Answer from the drawing. Dimensions are ordinates in mm from the lowest x, y and z of the part. A direction names the side the tool comes from. Coordinates: 2 decimals unless noted, no trailing zeros. Order: outer loops, then holes, each group sorted by start corner. A loop starts at its lowest first (then second) coordinate and runs counter-clockwise, first axis right, second up. Notation, with made-up numbers: (15.25, 30) - (66.25, 30) arc R14 cw to (66.25, 46) - close; hole circle Ø5 at (-22.5, 71.5). An arc over 180 degrees is marked (long way). Use a Markdown table: item, result. Add a question column.
Item 1: The part is cut by section A-A, the plane x = 60. Give the vertices of the cut face in (y, z) (1 decimal), then the cut area to 3 significant figures.
Item 2: The part is cut by section C-C, the plane z = 29.5. Give the vertices of the cut face in (x, y) (1 decimal).
Item 3: For the marked faces 1 and 2, determine the directions among +Z, -Z, +X, -X, +Y, -Y from which every point of the face is accessible in a straight line to the end or side of a thin tool.
Item 4: Find the intervals of material crossed by line 1 along Z through (x, y) = (42, 24); line 2 along Y through (x, z) = (83, 39.5) (1 decimal); line 3 along Y through (x, z) = (68.5, 32) (1 decimal), in increasing order.
Item 5: The part is cut by section D-D, the plane y = 98. Give the vertices of the cut face in (x, z), then the cut area to 3 significant figures.
Item 6: The part is cut by section B-B, the plane y = 57.5. Give the vertices of the cut face in (x, z).
Item 7: Flat-ended cylindrical pins translate along their axes: P1, Ø1, axis at x = 36, y = 64, coming from the -Z side; P2, Ø8, axis at x = 20, y = 32.5, coming from the +Z side. Find the tip coordinate at first contact, or state that the pin passes through.
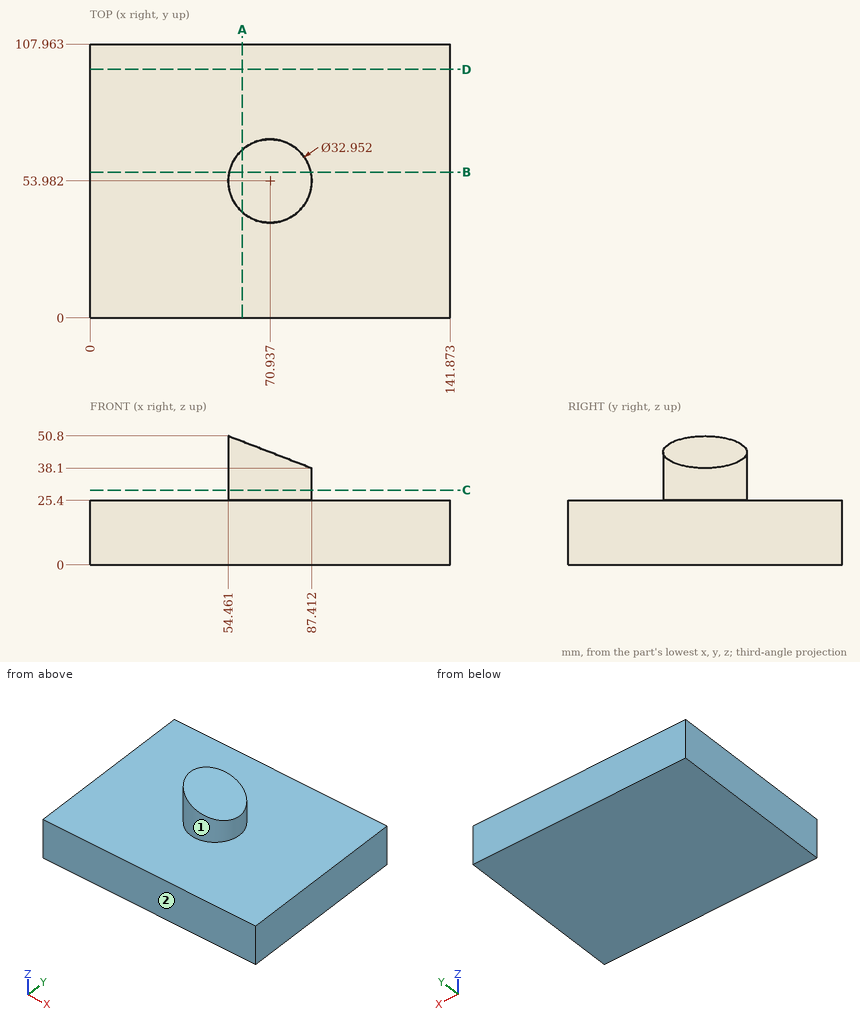
Solution:
| question | item | result |
|---|---|---|
| 1 | outline | (0, 0) - (108, 0) - (108, 25.4) - (66.3, 25.4) - (66.3, 48.7) - (41.7, 48.7) - (41.7, 25.4) - (0, 25.4) - close |
| 1 | area | 3,320 mm2 |
| 2 | outline | circle Ø33 at (70.9, 54) |
| 3 | face 1 | +Z |
| 3 | face 2 | +Z, -Z, +X, -X, -Y |
| 4 | line 1 | z = 0 to 25.4 |
| 4 | line 2 | y = 42.8 to 65.2 |
| 4 | line 3 | y = 37.7 to 70.3 |
| 5 | outline | (0, 0) - (141.87, 0) - (141.87, 25.4) - (0, 25.4) - close |
| 5 | area | 3,600 mm2 |
| 6 | outline | (0, 0) - (141.87, 0) - (141.87, 25.4) - (87.03, 25.4) - (87.03, 38.25) - (54.84, 50.65) - (54.84, 25.4) - (0, 25.4) - close |
| 7 | P1 | stops at z = 0 |
| 7 | P2 | stops at z = 25.4 |
